Design review of the part built by this model. Coordinates are the model's own, in mm. A direction names the side the tool comes from. Coordinates: 2 decimals unless noted, no trailing zeros. Write each loop counter-clockwise with the first axis right and the second up, starting at its lowest first coordinate (ties: lowest second). Pieces come first, ordered by that corner, then holes. Notation, with made-up numbers: M 11.25,-4 L 66.25,-4 A27 cw 66.25,28 Z; hole C 45,-22 d1. An arc over 180 degrees is marked long. Write item = value, one per line.
```python
from build123d import *

# Parameters (mm, degrees)
EXTRUDE_THIN1_DEPTH = 259
CUT_EXTRUDE1_DEPTH  = 260.926912804


with BuildPart() as part:
    # Sketch1 → Extrude-Thin1 (new body)
    with BuildSketch(Plane.XY):
        Polygon((15, 0), (0, 0), (0, 15), (-1, 15), (-1, -1), (15, -1), align=None)
    extrude(amount=EXTRUDE_THIN1_DEPTH)

    # Sketch2 → Cut-Extrude1 (cut, through all)
    with BuildSketch(Plane(origin=(0, -1, 0), x_dir=(-1, 0, 0), z_dir=(0, -1, 0))):
        Polygon((1, -259), (-15, -241), (-15, -259), align=None)
    extrude(amount=-CUT_EXTRUDE1_DEPTH, mode=Mode.SUBTRACT)


solid = part.part
```
Q1. Consider section C-C, the plane y = 4.25. State the section outline as (x, z) points (3 decimals).
Check result:
outline = M -1,0 L 0,0 L 0,257.875 L -1,259 Z
Q2. Machinability: for faces 1 (the flat face through (7, -1, 128)), 2 (the flat face through (8, 0, 127)), which of the approach directions +Z, -Z, +X, -X, +Y, -Y give a long, thin tool a straight path to every point of the face, cutting with its end or side? Answer none if there is none.
Check result:
face_1 = +Z, -Z, +X, -X, -Y
face_2 = +Z, -Z, +X, +Y
Q3. Consider section B-B, the plane x = 7. State the section outline as (y, z) points, and give its area (3 significant figures).
Check result:
outline = M -1,0 L 0,0 L 0,250 L -1,250 Z
area = 250 mm²
Q4. For P1, Ø7.5, axis at x = 10, z = 169.5, coming from the +Y side; P2, Ø7.5, axis at y = 10, z = 80.5, coming from the +X side, all flat-tipped, find the tip position at first contact; note any pin that passes through.
Check result:
P1 = 0
P2 = 0
Q5. Consider section A-A, the plane z = 131. State the section outline as (x, y) points, and give its area (3 significant figures).
Check result:
outline = M -1,-1 L 15,-1 L 15,0 L 0,0 L 0,15 L -1,15 Z
area = 31.0 mm²
Q6. Wall thickness on line 1 (Y direction, x = 5, z = 241.5); line 2 (Z direction, x = -0.25, y = 9): over which ranges is each line inside the solid? List them lowest first.
Check result:
line_1 = -1 to 0
line_2 = 0 to 258.16
